For this review, take the finished solid that the model builds, in its own axes (mm). A direction names the side the tool comes from. Give positions to 0.01 mm unless a question says otherwise; leave off trailing zeros. Loops run counter-clockwise (first coordinate to the right, second up) from the corner with the lowest first, then second, coordinate; pieces in that order, holes last. Notation, with made-up numbers: (-40, 23) -> (13, 23) arc R20 ccw to (13, 35) -> close; hole circle Ø4 at (13, 83). An arc over 180 degrees is marked (long way). One line per question, with ' | ' between items. Start each with the question number.
(1) Consider section A-A (x = 1.75). Write out the cut boundary in (y, z).
(2) Insertion check: P1, Ø2, axis at x = 4.5, z = -2, coming from the +Y side; P2, Ø6, axis at y = 28.39, z = 0, coming from the +X side; P3, Ø8, axis at x = -5, y = 17, coming from the -Z side. Each pin has a flat end and moves straight along its axis. Give the tip position at first contact, or say it passes through.
(3) Consider section C-C (y = 5.5). Write out the cut boundary in (x, z).
(4) Consider section D-D (x = -4.75). Write out the cut boundary in (y, z).
(5) Wall thickness on probe 1 along X at (y, z) = (2, 0); probe 2 along X at (y, z) = (28, 3); probe 3 along Z at (x, y) = (0.5, 22): over which ranges is each line inside the solid? List them lowest first.
(6) Consider section B-B (z = 1). Write out the cut boundary in (x, y), and give its area (3 significant figures).
(7) Tool access review of faces 5 (the flat face through (-4, 10, 0)), 6 (the cylindrical face through (0.33, 4.93, -7.493)), 7 (the flat face through (0, 19, -7.071)), 8 (the cylindrical face through (1.88, 3.7, -5.96)), 9 (the flat face through (4, 10, 0)): name each direction out of +Z, -Z, +X, -X, +Y, -Y from which nothing blocks a thin tool from reaching the whole face with its end or side.
(8) Draft analysis for pull direction X (two halves, no side actions). For faces 1 (the flat face through (-2.5, 22, 0)), 2 (the flat face through (2.5, 22, 0)), 3 (the flat face through (0, 7.5, 0)), 4 (the flat face through (0, 19, 7.071)), state which applies: +X half, -X half, draft (parallel to the pull), parting line (faces both ways), or undercut.
from build123d import *

# Parameters (mm, degrees)
SKETCH1_R           = 7.5
BOSS_EXTRUDE1_DEPTH = 10
SKETCH2_R           = 6.25
CUT_EXTRUDE2_DEPTH  = 7.5
SKETCH3_W           = 5
SKETCH3_H           = 14.142135624
BOSS_EXTRUDE2_DEPTH = 25
SKETCH4_R           = 2.5
CUT_EXTRUDE3_DEPTH  = 5
FILLET1_R           = 7.65


with BuildPart() as part:
    # Sketch1 → Boss-Extrude1 (new body)
    with BuildSketch(Plane(origin=(0, 0, 0), x_dir=(1, 0, 0), z_dir=(0, 1, 0))):
        with Locations(Location((0, 0, 0), (0, 0, 270))):
            Circle(SKETCH1_R)
    extrude(amount=BOSS_EXTRUDE1_DEPTH)

    # Sketch2 → Cut-Extrude2 (cut)
    with BuildSketch(Plane.XZ):
        with Locations(Location((0, 0, 0), (0, 0, 270))):
            Circle(SKETCH2_R)
    extrude(amount=-CUT_EXTRUDE2_DEPTH, mode=Mode.SUBTRACT)

    # Sketch3 → Boss-Extrude2 (add)
    with BuildSketch(Plane(origin=(0, 10, 0), x_dir=(1, 0, 0), z_dir=(0, 1, 0))):
        Rectangle(SKETCH3_W, SKETCH3_H)
    extrude(amount=BOSS_EXTRUDE2_DEPTH)

    # Sketch4 → Cut-Extrude3 (cut)
    with BuildSketch(Plane(origin=(2.5, 0, 0), x_dir=(0, 0, -1), z_dir=(1, 0, 0))):
        with Locations((0, 28.391835492)):
            Circle(SKETCH4_R)
    extrude(amount=-CUT_EXTRUDE3_DEPTH, mode=Mode.SUBTRACT)

    # Fillet1
    # the kernel refuses this fillet: 7.65 mm, written as the material it takes off along each edge
    with BuildSketch(Plane(origin=(21.625, 35, -7.071067812), x_dir=(0, -1, 0), z_dir=(-1, 0, 0)), Plane(origin=(-21.625, 35, 7.071067812), x_dir=(0, -1, 0), z_dir=(1, 0, 0))) as fillet1_piece_1:
        with BuildLine():
            CenterArc((FILLET1_R, FILLET1_R), FILLET1_R, 180, 90)
            Line((0, FILLET1_R), (0, 0))
            Line((0, 0), (FILLET1_R, 0))
        make_face()
    extrude(amount=43.25, mode=Mode.SUBTRACT)


solid = part.part
A:
1) outline: (0, -7.29) -> (10, -7.29) -> (10, -7.07) -> (27.35, -7.07) arc R7.65 ccw to (34.98, 0) arc R7.65 ccw to (27.35, 7.07) -> (10, 7.07) -> (10, 7.29) -> (0, 7.29) -> (0, 6) -> (7.5, 6) -> (7.5, -6) -> (0, -6) -> close; hole circle Ø5 at (28.39, 0)
2) P1: stops at y = 10 | P2: stops at x = 2.5 | P3: stops at z = -7.07
3) outline: circle Ø15 at (0, 0); hole circle Ø12.5 at (0, 0)
4) outline: (0, -5.8) -> (10, -5.8) -> (10, 5.8) -> (0, 5.8) -> (0, 4.06) -> (7.5, 4.06) -> (7.5, -4.06) -> (0, -4.06) -> close
5) probe 1: x = -7.5 to -6.25, 6.25 to 7.5 | probe 2: x = -2.5 to 2.5 | probe 3: z = -7.07 to 7.07
6) outline: (-7.43, 0) -> (-6.17, 0) -> (-6.17, 7.5) -> (6.17, 7.5) -> (6.17, 0) -> (7.43, 0) -> (7.43, 10) -> (2.5, 10) -> (2.5, 26.1) -> (-2.5, 26.1) -> (-2.5, 10) -> (-7.43, 10) -> close; (-2.5, 30.68) -> (2.5, 30.68) -> (2.5, 34.84) -> (-2.5, 34.84) -> close | area: 157 mm^2
7) face 5: +Z, -Z, -X, +Y | face 6: +Y, -Y | face 7: -Z, +X, -X, +Y | face 8: -Y | face 9: +Z, -Z, +X, +Y
8) face 1: -X half | face 2: +X half | face 3: undercut | face 4: draft
